Geometry check sheet. Reference: drawing and pictorial views, mm from the part's lowest x, y, z. Give positions to 0.01 mm unless a question says otherwise; leave off trailing zeros. Loops run counter-clockwise (first coordinate to the right, second up) from the corner with the lowest first, then second, coordinate; pieces in that order, holes last. Notation, with made-up numbers: (65.25, 2) - (122.25, 2) arc R24 cw to (122.25, 21) - close; hole circle Ø6 at (10, 13). An arc over 180 degrees is marked (long way). Put each result on its own line as item: value. Start each with the question number.
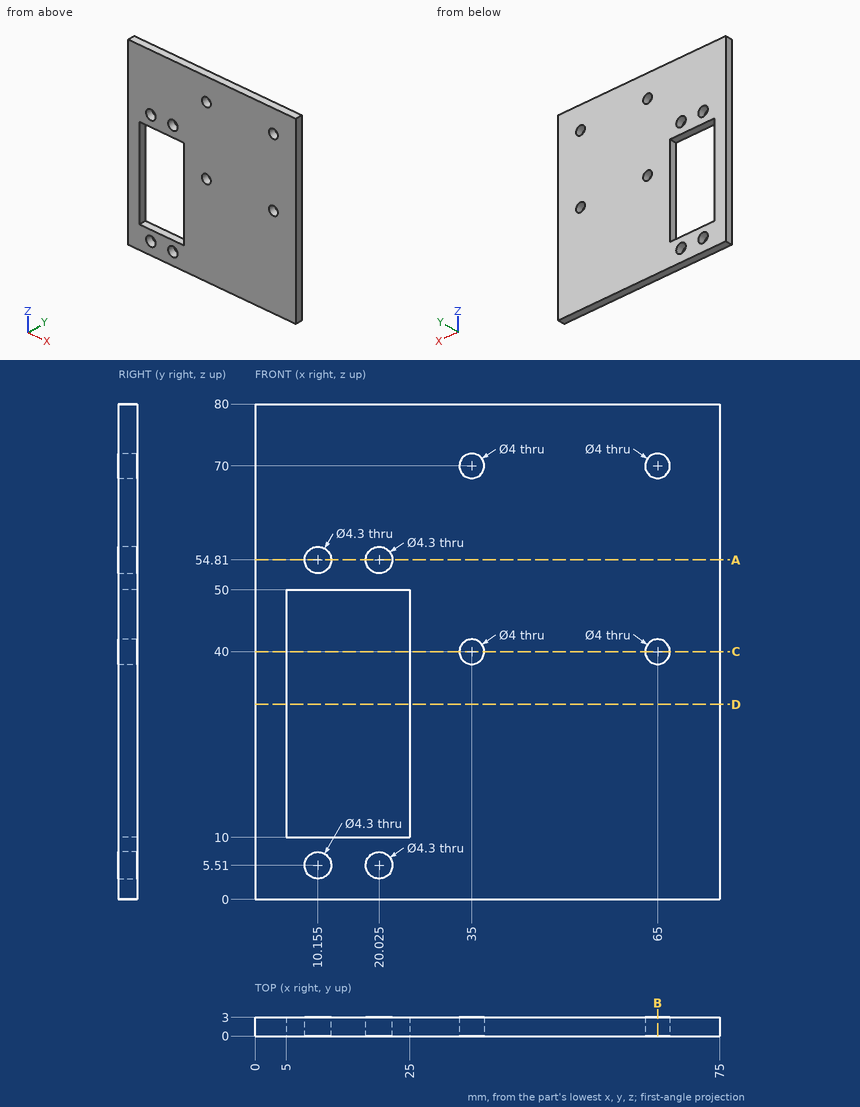
1) Section check A-A, the plane z = 54.81. Enter the section's corners in (x, y) (3 decimals).
2) Section check B-B, the plane x = 65. Enter the section's corners in (y, z), plus the area to 3 significant figures.
3) Section check C-C, the plane z = 40. Enter the section's corners in (x, y), plus the area to 3 significant figures.
4) Depth check by flat-ended pin: P1, Ø6.5, axis at x = 65, z = 40, coming from the +Y side. Enter the tip coordinate at first touch or a pass-through.
5) Scan lines: line 1 along X through (y, z) = (1, 40); line 2 along X through (y, z) = (2.3, 5.51) (3 decimals); line 3 along X through (y, z) = (0.9, 70). Record each from-to range of solid material in increasing order. Write a range as from..to.
6) Section check D-D, the plane z = 31.5. Enter the section's corners in (x, y), plus the area to 3 significant figures.
Results are:
1. outline: (0, 0) - (8.005, 0) - (8.005, 3) - (0, 3) - close; (12.305, 0) - (17.875, 0) - (17.875, 3) - (12.305, 3) - close; (22.175, 0) - (75, 0) - (75, 3) - (22.175, 3) - close
2. outline: (0, 0) - (3, 0) - (3, 38) - (0, 38) - close; (0, 42) - (3, 42) - (3, 68) - (0, 68) - close; (0, 72) - (3, 72) - (3, 80) - (0, 80) - close
2. area: 216 mm2
3. outline: (0, 0) - (5, 0) - (5, 3) - (0, 3) - close; (25, 0) - (33, 0) - (33, 3) - (25, 3) - close; (37, 0) - (63, 0) - (63, 3) - (37, 3) - close; (67, 0) - (75, 0) - (75, 3) - (67, 3) - close
3. area: 141 mm2
4. P1: stops at y = 3
5. line 1: x = 0..5, 25..33, 37..63, 67..75
5. line 2: x = 0..8.005, 12.305..17.875, 22.175..75
5. line 3: x = 0..33, 37..63, 67..75
6. outline: (0, 0) - (5, 0) - (5, 3) - (0, 3) - close; (25, 0) - (75, 0) - (75, 3) - (25, 3) - close
6. area: 165 mm2
